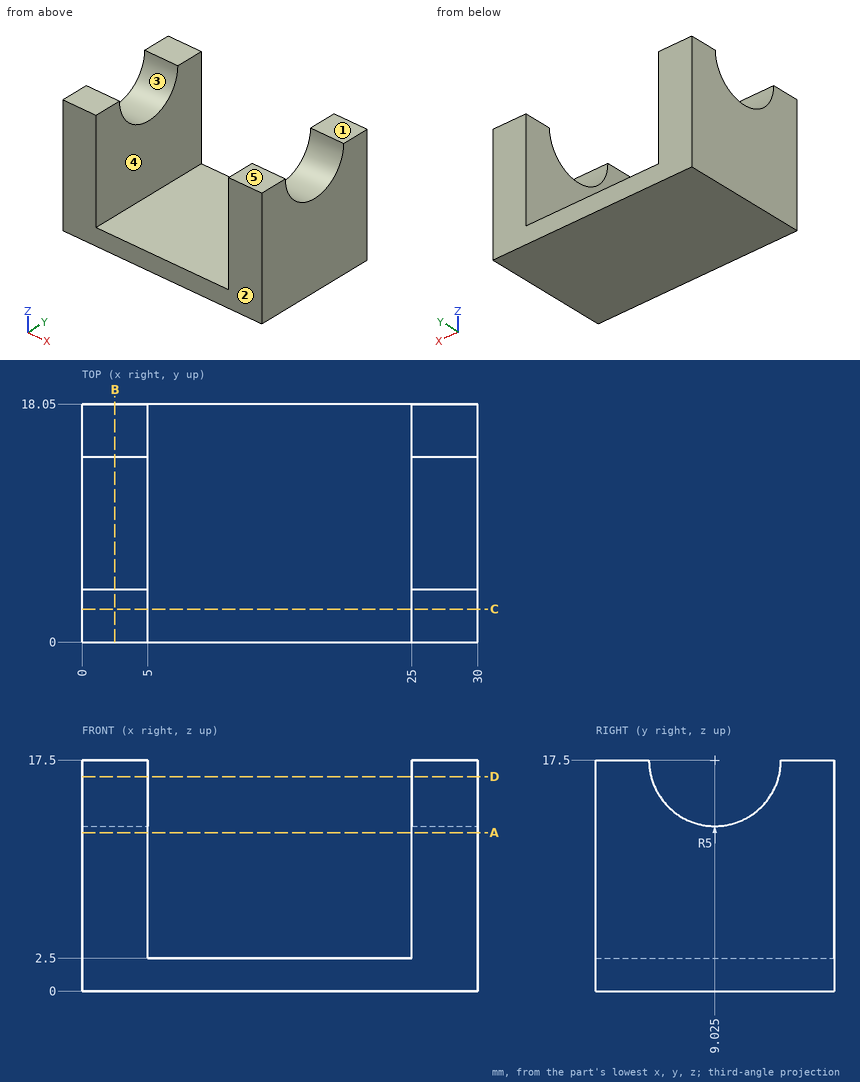
Part print with two shaded views. Sizes in mm from the minimum x, y, z corner. A direction names the side the tool comes from. Round coordinates to 2 decimals unless told otherwise and drop trailing zeros. Order: outer loops, then holes, each group sorted by start corner. A loop starts at its lowest first (then second) coordinate and runs counter-clockwise, first axis right, second up.
(1) Band-saw the part on B-B (x = 2.5). List the corners of the cut face in (y, z) (3 decimals).
(2) 3-axis set-ups, long thin cutter, end or side, ignore diameter. For the marked faces 4 and 5: which of +Z, -Z, +X, -X, +Y, -Y reach the whole face in a straight line?
(3) Band-saw the part on C-C (y = 2.5). List the corners of the cut face in (x, z).
(4) Pin check, flat tips, straight feed: pin 1 (1.5 mm diameter, centred on x = 5.5, y = 7.5, fed in from +Z) (3 decimals); pin 2 (4 mm diameter, centred on x = 16.5, y = 12, fed in from +Z); pin 3 (6 mm diameter, centred on x = 4.5, y = 9, fed in from +Z). Stop position of each tip, or through.
(5) Band-saw the part on D-D (z = 16.25). List the corners of the cut face in (x, y), then the cut area to 3 significant figures.
(6) Drill centre lines: line 1 (X direction, y = 16.25, z = 8.25); line 2 (Z direction, x = 19, y = 13.5); line 3 (Z direction, x = 2.25, y = 13.5). Where is each one in solid material? Low to high.
(7) Pull direction Y, two halves, no side cores. Call the marked faces 1, 2 and 3: released by +Y, released by -Y, zero draft, split by the parting line, or undercut.
(8) Band-saw the part on A-A (z = 12). List the corners of the cut face in (x, y), then the cut area to 4 significant figures.
Verdict:
1. outline: (0, 0) - (18.05, 0) - (18.05, 17.5) - (14.025, 17.5) arc R5 cw to (4.025, 17.5) - (0, 17.5) - close
2. face 4: +Z, +Y, -Y
2. face 5: +Z, +X, -X, +Y, -Y
3. outline: (0, 0) - (30, 0) - (30, 17.5) - (25, 17.5) - (25, 2.5) - (5, 2.5) - (5, 17.5) - (0, 17.5) - close
4. pin 1: stops at z = 12.955
4. pin 2: stops at z = 2.5
4. pin 3: stops at z = 13.52
5. outline: (0, 0) - (5, 0) - (5, 4.18) - (0, 4.18) - close; (0, 13.87) - (5, 13.87) - (5, 18.05) - (0, 18.05) - close; (25, 0) - (30, 0) - (30, 4.18) - (25, 4.18) - close; (25, 13.87) - (30, 13.87) - (30, 18.05) - (25, 18.05) - close
5. area: 83.7 mm2
6. line 1: x = 0 to 5, 25 to 30
6. line 2: z = 0 to 2.5
6. line 3: z = 0 to 15.27
7. face 1: zero draft
7. face 2: released by -Y
7. face 3: undercut
8. outline: (0, 0) - (5, 0) - (5, 18.05) - (0, 18.05) - close; (25, 0) - (30, 0) - (30, 18.05) - (25, 18.05) - close
8. area: 180.5 mm2
